from build123d import *

# Parameters (mm, degrees)
SKETCH1_R                = 8.73125
BOSS_EXTRUDE1_DEPTH      = 7.62
SKETCH3_R                = 8.7376
SKETCH3_R_2              = 3.27025
BOSS_EXTRUDE2_DEPTH      = 1.5875
BOSS_EXTRUDE2_DEPTH_BACK = 1.5875
SKETCH4_R                = 1.98374
CUT_EXTRUDE1_DEPTH       = 10.16


with BuildPart() as part:
    # Sketch1 → Boss-Extrude1 (new body)
    with BuildSketch(Plane.XY):
        with BuildLine():
            Line((4.5, 4.699), (-4.5, 4.699))
            Line((-4.5, 4.699), (-4.5, 0))
            Line((-4.5, 0), (-19.05, 0))
            Line((-19.05, 0), (-19.05, 9.36625))
            Line((-19.05, 9.36625), (-12.54125, 15.875))
            ThreePointArc((-12.54125, 15.875), (0, 28.41625), (12.54125, 15.875))
            Line((12.54125, 15.875), (19.05, 9.36625))
            Line((19.05, 9.36625), (19.05, 0))
            Line((19.05, 0), (4.5, 0))
            Line((4.5, 0), (4.5, 4.699))
        make_face()
        with Locations((0, 15.875)):
            Circle(SKETCH1_R, mode=Mode.SUBTRACT)
    extrude(amount=BOSS_EXTRUDE1_DEPTH)

    # Sketch3 → Boss-Extrude2 (add, two sides)
    with BuildSketch(Plane.XY.offset(3.81)) as boss_extrude2_sk:
        with Locations((0, 15.875)):
            Circle(SKETCH3_R)
        with Locations((0, 15.875)):
            Circle(SKETCH3_R_2, mode=Mode.SUBTRACT)
    extrude(amount=BOSS_EXTRUDE2_DEPTH)
    extrude(boss_extrude2_sk.sketch, amount=-BOSS_EXTRUDE2_DEPTH_BACK)

    # Sketch4 → Cut-Extrude1 (cut)
    with BuildSketch(Plane(origin=(0, 0, 0), x_dir=(-1, 0, 0), z_dir=(0, -1, 0))):
        with Locations((-11.43, -3.81)):
            Circle(SKETCH4_R)
        with Locations((11.43, -3.81)):
            Circle(SKETCH4_R)
    extrude(amount=-CUT_EXTRUDE1_DEPTH, mode=Mode.SUBTRACT)


solid = part.part
Part model, mm, in its own coordinate system. A direction names the side the tool comes from. Coordinates: 2 decimals unless noted, no trailing zeros. Write each loop counter-clockwise with the first axis right and the second up, starting at its lowest first coordinate (ties: lowest second). Pieces come first, ordered by that corner, then holes. Notation, with made-up numbers: M -22.5,-31.5 L -4.5,-31.5 A20 cw -4.5,-2.5 Z; hole C 12,25 d4. An arc over 180 degrees is marked long. Return JSON: item names as keys, results as strings.
1. Saw through at A-A, the plane y = 4.25. Write the cut outline in (x, z).
Determined:
{"outline": "M -19.05,0 L -4.5,0 L -4.5,7.62 L -19.05,7.62 Z; M 4.5,0 L 19.05,0 L 19.05,7.62 L 4.5,7.62 Z; hole C -11.43,3.81 d3.97; hole C 11.43,3.81 d3.97"}
2. Flat gauge pins, fed straight in: pin 1 Ø10.5 at (x, y) = (0, 15.875) entering from -Z; pin 2 Ø4 at (x, z) = (2, 2) entering from -Y; pin 3 Ø10.5 at (x, y) = (0, 15.875) entering from +Z. Where does each tip first touch, or does it go through?
Determined:
{"pin 1": "z = 2.22", "pin 2": "y = 4.7", "pin 3": "z = 5.4"}
3. Saw through at B-B, the plane x = 0. Write the cut outline in (y, z).
Determined:
{"outline": "M 4.7,0 L 7.14,0 L 7.14,2.22 L 12.6,2.22 L 12.6,5.4 L 7.14,5.4 L 7.14,7.62 L 4.7,7.62 Z; M 19.15,2.22 L 24.61,2.22 L 24.61,0 L 28.42,0 L 28.42,7.62 L 24.61,7.62 L 24.61,5.4 L 19.15,5.4 Z"}
4. Pull direction Y, two halves, no side cores. Call faces 5 (the face through (-1.89, 7.35, 6.49)), 6 (the face through (-0.276, 28.413, 3.757)), 7 (the face through (-19.05, 5, 4)), 8 (the face through (-1.89, 7.35, 1.1)): pulls with the +Y half, pulls with the -Y half, needs draft (parallel to the pull), parting line crosses it, or undercut.
Determined:
{"face 5": "undercut", "face 6": "pulls with the +Y half", "face 7": "needs draft", "face 8": "undercut"}
5. Probe L1, parallel to Z at x = 11.43, y = 7.25; L2, parallel to X at y = 3, z = 3.81; L3, parallel to X at y = 4, z = 4.5. List the from-to ranges inside material, lowest first.
Determined:
{"L1": "0 to 1.83, 5.79 to 7.62", "L2": "-19.05 to -13.41, -9.45 to -4.5, 4.5 to 9.45, 13.41 to 19.05", "L3": "-19.05 to -13.29, -9.57 to -4.5, 4.5 to 9.57, 13.29 to 19.05"}
6. 3-axis set-ups, long thin cutter, end or side, ignore diameter. For faces 1 (the face through (0, 12, 2.222)), 2 (the face through (-4.5, 2, 4)), 3 (the face through (0, 12, 5.398)), 4 (the face through (-13.32, 5.01, 3.21)): which of +Z, -Z, +X, -X, +Y, -Y reach the whole face in a straight line?
Determined:
{"face 1": "-Z", "face 2": "+Z, -Z, -Y", "face 3": "+Z", "face 4": "-Y"}
7. Saw through at D-D, the plane y = 13.25. Write the cut outline in (x, z).
Determined:
{"outline": "M -15.17,0 L -8.33,0 L -8.33,2.22 L -1.95,2.22 L -1.95,5.4 L -8.33,5.4 L -8.33,7.62 L -15.17,7.62 Z; M 1.95,2.22 L 8.33,2.22 L 8.33,0 L 15.17,0 L 15.17,7.62 L 8.33,7.62 L 8.33,5.4 L 1.95,5.4 Z"}
